Part print with two shaded views. Sizes in mm from the minimum x, y, z corner. Coordinates: 2 decimals unless noted, no trailing zeros.
Q1. Drill centre lines: probe 1 along X at (y, z) = (12.75, 26.5) (1 decimal); probe 2 along X at (y, z) = (12.75, 219) (1 decimal); probe 3 along Z at (x, y) = (283, 16.75) (1 decimal). Where is each one in solid material? Low to high.
Q2. Pin check, flat tips, straight feed: P1, Ø6, axis at x = 245, z = 65, coming from the -Y side; P2, Ø1.8, axis at x = 122, z = 33, coming from the +Y side. Stop position of each tip, or through.
Q3. Band-saw the part on A-A, the plane y = 9.25. State how many separate pieces and enclosed holes the cut face has, plus the area to 3 significant figures.
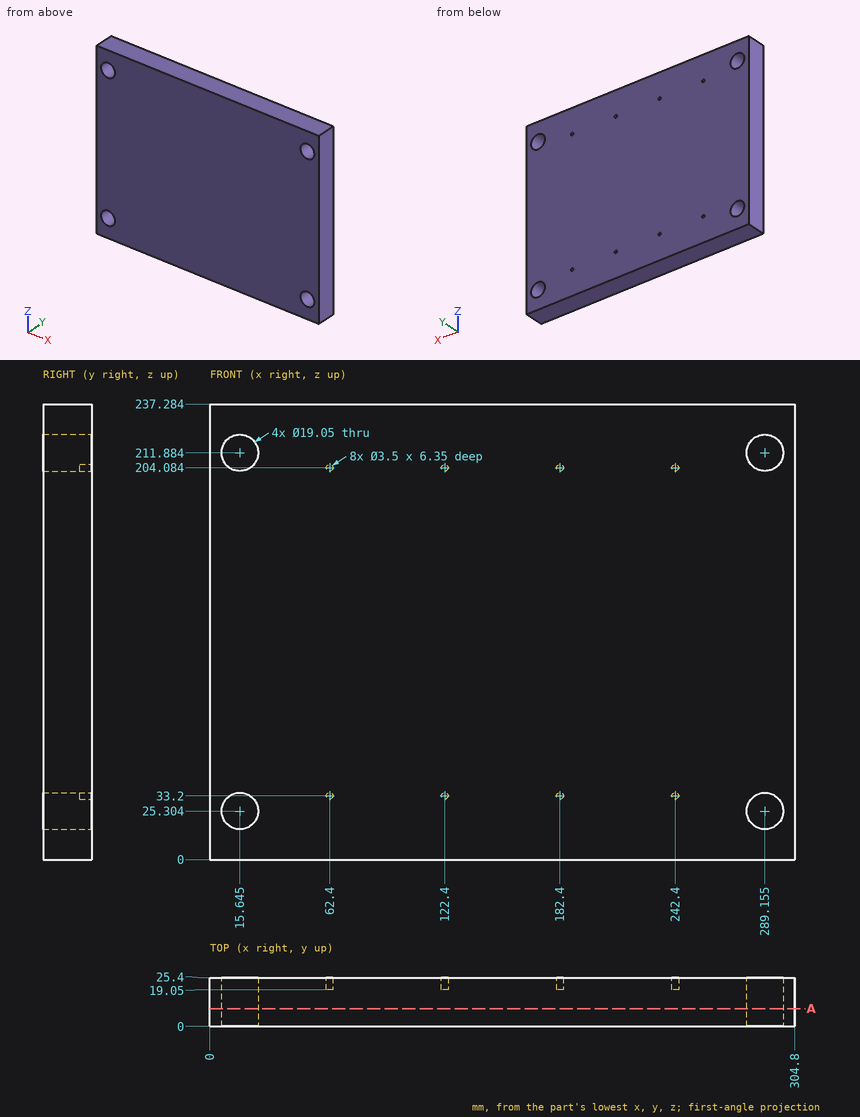
Answer sheet:
1. probe 1: x = 0 to 6.2, 25.1 to 279.7, 298.6 to 304.8
1. probe 2: x = 0 to 9.3, 22 to 282.8, 295.5 to 304.8
1. probe 3: z = 0 to 18, 32.6 to 204.6, 219.2 to 237.3
2. P1: stops at y = 0
2. P2: stops at y = 19.05
3. separate pieces: 1
3. enclosed holes: 4
3. area: 71,200 mm2
